Autodesk Inventor part; units mm, degrees
ref_plane "YZ Plane" through (0, 0, 0) normal (1, 0, 0) x (0, 1, 0)
ref_plane "XZ Plane" through (0, 0, 0) normal (0, 1, 0) x (-1, 0, 0)
ref_plane "XY Plane" through (0, 0, 0) normal (0, 0, 1) x (1, 0, 0)
sketch "Esboço1" plane through (0, 0, 0) normal (0, 1, 0) x (-1, 0, 0)
  line L0 (0, -4.5815) -> (-2.9062, -6.2522)
  line L1 (-2.9062, -6.2522) -> (-5.8062, -4.5707)
  line L2 (-5.8062, -4.5707) -> (-5.8, -1.2185)
  line L3 (-5.8, -1.2185) -> (-2.8938, 0.4522)
  line L4 (-2.8938, 0.4522) -> (0.0062, -1.2293)
  line L5 (0.0062, -1.2293) -> (0, -4.5815)
  circle A0 centre (-2.9, -2.9) radius 1.5
  point P0 (0, 0)
  dimension "d11" = 3
extrude "Extrusão1" add sketch "Esboço1" along normal blind 2.5
properties part number "Porca M3"
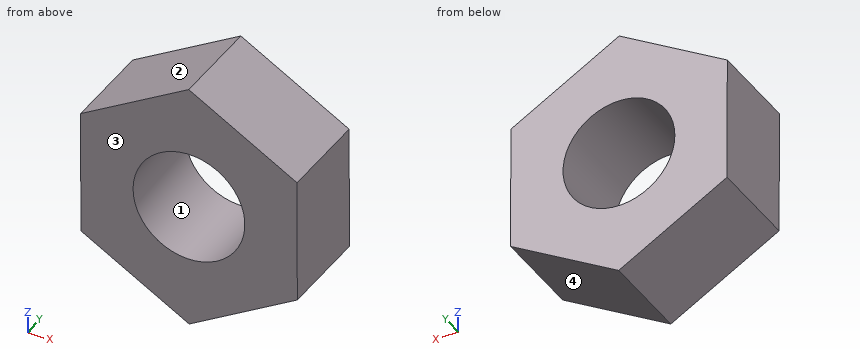
The model under review builds one solid part; all positions refer to its coordinate system, in mm. Face numbers are marked on the shaded views. Round coordinates to 2 decimals unless told otherwise and drop trailing zeros. Write each loop counter-clockwise with the first axis right and the second up, starting at its lowest first coordinate (ties: lowest second). Pieces come first, ordered by that corner, then holes. Notation, with made-up numbers: M 17,21.25 L 76,21.25 A16 ccw 76,48.25 Z; hole C 59,46.5 d2. An arc over 180 degrees is marked long. Use a Markdown table: item, result. Add a question column.
Q1. To check wall thickness, follow line 1 (Z direction, x = 3.75, y = 1.3); line 2 (X direction, y = 0.1, z = -4.5); line 3 (Z direction, x = 2.15, y = 2.35). State the ranges of each line that lie inside material, in increasing order.
Q2. We need section C-C, the plane z = -3.5. State the section outline as (x, y) points.
Q3. We need section D-D, the plane x = 0.6. State the section outline as (y, z) points, plus the area to 3 significant figures.
Q4. We need section B-B, the plane x = 3.15. State the section outline as (y, z) points, plus the area to 3 significant figures.
Q5. We need section A-A, the plane y = 1.3. State the section outline as (x, z) points.
Q6. The part is to be moulded in two halves that separate along Z. For the marked faces 1, 2, 3 and 4, say which applies: pulls with the +Z half, pulls with the -Z half, needs draft (parallel to the pull), parting line crosses it, or undercut.
Findings below:
| question | item | result |
|---|---|---|
| 1 | line 1 | z = -5.76 to -4.14, -1.66 to -0.04 |
| 1 | line 2 | x = 0 to 5.81 |
| 1 | line 3 | z = -5.82 to -4.2, -1.6 to 0.02 |
| 2 | outline | M 0,0 L 1.53,0 L 1.53,2.5 L 0,2.5 Z; M 4.27,0 L 5.8,0 L 5.8,2.5 L 4.27,2.5 Z |
| 3 | outline | M 0,-4.93 L 2.5,-4.93 L 2.5,-0.88 L 0,-0.88 Z |
| 3 | area | 10.1 mm² |
| 4 | outline | M 0,-6.11 L 2.5,-6.11 L 2.5,-4.38 L 0,-4.38 Z; M 0,-1.42 L 2.5,-1.42 L 2.5,0.3 L 0,0.3 Z |
| 4 | area | 8.64 mm² |
| 5 | outline | M -0.01,-1.23 L 0,-4.58 L 2.91,-6.25 L 5.81,-4.57 L 5.8,-1.22 L 2.89,0.45 Z; hole C 2.9,-2.9 d3 |
| 6 | face 1 | undercut |
| 6 | face 2 | pulls with the +Z half |
| 6 | face 3 | needs draft |
| 6 | face 4 | pulls with the -Z half |
